Could you check a few things on this model? Use its own coordinates, in mm. A direction names the side the tool comes from. Coordinates: 2 decimals unless noted, no trailing zeros. Loops run counter-clockwise (first coordinate to the right, second up) from the corner with the lowest first, then second, coordinate; pieces in that order, holes last.
1) Imagine slicing it at C-C on y = 2.3. Please give me the cut outline in (x, z) (3 decimals), plus the area to 3 significant figures.
2) If I drill on line 1 along Z through (x, y) = (7, 2.3); line 2 along X through (y, z) = (3.9, -5); line 3 along X through (y, z) = (3.65, 4), over which ranges is the centre line in solid material (lowest first)?
3) Imagine slicing it at D-D on x = -17. Please give me the cut outline in (y, z).
4) Imagine slicing it at B-B on x = 0. Please give me the cut outline in (y, z), plus the area to 3 significant figures.
5) For faces 1 (the face through (20, 2, 32.5)), 2 (the face through (-20, 2, 32.5)), 3 (the face through (0, 3, -2.5)), which set-ups out of +Z, -Z, +X, -X, +Y, -Y let a thin tool reach every point of the face, with its end or its side?
6) Thinking about a two-plate mould opening in Z: for faces 4 (the face through (-30, 2, 0)), 5 (the face through (0.66, 2.465, -62.493)), 6 (the face through (-5.23, 2.46, -49.31)), 7 (the face through (0, 2, 41.5)), which applies, released by +Z, released by -Z, zero draft, split by the parting line, or undercut?
7) Will these pins go through, and if not, where does the flat tip stop? P1, Ø3, axis at y = 3.5, z = -51, coming from the +X side; P2, Ø5.5, axis at x = -4.78, z = 2.16, coming from the +Y side; P3, Ø3.5, axis at x = -4.78, z = -47.26, coming from the +Y side; P4, Ø2.5, axis at y = 3.5, z = 36.5, coming from the +X side.
8) Imagine slicing it at A-A on z = -26.5. Please give me the cut outline in (x, y), plus the area to 3 significant figures.
```python
from build123d import *

# Parameters (mm, degrees)
SKETCH1_W               = 60
SKETCH1_H               = 65
SKETCH1_W_2             = 20
SKETCH1_H_2             = 9
BOSS_EXTRUDE1_DEPTH     = 5
SKETCH2_W               = 20
SKETCH2_H               = 40
CUT_EXTRUDE1_DEPTH      = 6
SKETCH3_R               = 2.1
CUT_EXTRUDE2_DEPTH      = 1
CUT_EXTRUDE2_DEPTH_BACK = 6


with BuildPart() as part:
    # Sketch1 → Boss-Extrude1 (new body)
    with BuildSketch(Plane(origin=(0, 0, 0), x_dir=(1, 0, 0), z_dir=(0, 1, 0))):
        Rectangle(SKETCH1_W, SKETCH1_H)
        with Locations((0, -37)):
            Rectangle(SKETCH1_W_2, SKETCH1_H_2)
        with BuildLine():
            Line((-30, 32.5), (30, 32.5))
            ThreePointArc((30, 32.5), (0, 62.5), (-30, 32.5))
        make_face()
    extrude(amount=BOSS_EXTRUDE1_DEPTH)

    # Sketch2 → Cut-Extrude1 (cut, through all)
    with BuildSketch(Plane(origin=(0, 5, 0), x_dir=(1, 0, 0), z_dir=(0, 1, 0))):
        with Locations((0, 22.5)):
            Rectangle(SKETCH2_W, SKETCH2_H)
    extrude(amount=-CUT_EXTRUDE1_DEPTH, mode=Mode.SUBTRACT)

    # Sketch3 → Cut-Extrude2 (cut, two sides)
    with BuildSketch(Plane.XZ) as cut_extrude2_sk:
        with Locations((-4.775, 2.161145618)):
            Circle(SKETCH3_R)
        with Locations((5.075, 2.161145618)):
            Circle(SKETCH3_R)
        with Locations((5.075, -47.261145618)):
            Circle(SKETCH3_R)
        with Locations((-4.775, -47.261145618)):
            Circle(SKETCH3_R)
    extrude(amount=CUT_EXTRUDE2_DEPTH, mode=Mode.SUBTRACT)
    extrude(cut_extrude2_sk.sketch, amount=-CUT_EXTRUDE2_DEPTH_BACK, mode=Mode.SUBTRACT)


solid = part.part
```
Filled in:
1. outline: (-30, -32.5) arc R30 ccw to (30, -32.5) - (30, 32.5) - (10, 32.5) - (10, 41.5) - (-10, 41.5) - (-10, 32.5) - (-30, 32.5) - close; hole (-10, -42.5) - (10, -42.5) - (10, -2.5) - (-10, -2.5) - close; hole circle Ø4.2 at (-4.775, -47.261); hole circle Ø4.2 at (-4.775, 2.161); hole circle Ø4.2 at (5.075, -47.261); hole circle Ø4.2 at (5.075, 2.161)
1. area: 4,640 mm2
2. line 1: z = -61.67 to -48.1, -46.42 to -42.5, -2.5 to 1.32, 3 to 41.5
2. line 2: x = -30 to -10, 10 to 30
2. line 3: x = -30 to -5.79, -3.76 to 4.06, 6.09 to 30
3. outline: (0, -57.22) - (5, -57.22) - (5, 32.5) - (0, 32.5) - close
4. outline: (0, -62.5) - (5, -62.5) - (5, -42.5) - (0, -42.5) - close; (0, -2.5) - (5, -2.5) - (5, 41.5) - (0, 41.5) - close
4. area: 320 mm2
5. face 1: +Z, +X, +Y, -Y
5. face 2: +Z, -X, +Y, -Y
5. face 3: +Y, -Y
6. face 4: zero draft
6. face 5: released by -Z
6. face 6: undercut
6. face 7: released by +Z
7. P1: stops at x = 24.72
7. P2: stops at y = 5
7. P3: passes through
7. P4: stops at x = 10
8. outline: (-30, 0) - (-10, 0) - (-10, 5) - (-30, 5) - close; (10, 0) - (30, 0) - (30, 5) - (10, 5) - close
8. area: 200 mm2
